from build123d import *

# Parameters (mm, degrees)
SCHIZZO1_R                   = 3.5
ESTRUSIONE_ESTRUSIONE1_DEPTH = 3
ESTRUSIONE_ESTRUSIONE2_DEPTH = 1.5
SCHIZZO3_R                   = 2.5
TAGLIO_ESTRUSIONE1_DEPTH     = 2
RACCORDO1_R                  = 1
SKETCH2_R                    = 1
CUT_EXTRUDE1_DEPTH           = 17.046806536


with BuildPart() as part:
    # Schizzo1 → Estrusione-Estrusione1 (new body)
    with BuildSketch(Plane(origin=(0, 0, 0), x_dir=(1, 0, 0), z_dir=(0, 1, 0))):
        with Locations(Location((0, 0, 0), (0, 0, 270))):
            Circle(SCHIZZO1_R)
    extrude(amount=ESTRUSIONE_ESTRUSIONE1_DEPTH)

    # Schizzo2 → Estrusione-Estrusione2 (add)
    with BuildSketch(Plane(origin=(0, 3, 0), x_dir=(1, 0, 0), z_dir=(0, 1, 0))):
        with BuildLine():
            Line((15, 1.5), (15, -1.5))
            Line((15, -1.5), (0.469834495, -3.468321719))
            ThreePointArc((0.469834495, -3.468321719), (-3.5, 0), (0.469834495, 3.468321719))
            Line((0.469834495, 3.468321719), (15, 1.5))
        make_face()
    extrude(amount=ESTRUSIONE_ESTRUSIONE2_DEPTH)

    # Schizzo3 → Taglio-Estrusione1 (cut)
    with BuildSketch(Plane.XZ):
        with Locations(Location((0, 0, 0), (0, 0, 270))):
            Circle(SCHIZZO3_R)
    extrude(amount=-TAGLIO_ESTRUSIONE1_DEPTH, mode=Mode.SUBTRACT)

    # Raccordo1
    raccordo1_edges = [part.edges().sort_by_distance(p)[0] for p in [
        (15, 3.75, 1.5),
        (15, 3.75, -1.5),
    ]]
    fillet(raccordo1_edges, radius=RACCORDO1_R)

    # Sketch2 → Cut-Extrude1 (cut, through all)
    with BuildSketch(Plane(origin=(0, 4.5, 0), x_dir=(1, 0, 0), z_dir=(0, 1, 0))):
        with Locations(Location((13, 0.055401887, 0), (0, 0, 270))):
            Circle(SKETCH2_R)
    extrude(amount=-CUT_EXTRUDE1_DEPTH, mode=Mode.SUBTRACT)


solid = part.part
Work out the finished part from the listing and answer in its coordinate system (mm). A direction names the side the tool comes from. Round coordinates to 2 decimals unless told otherwise and drop trailing zeros. Write each loop counter-clockwise with the first axis right and the second up, starting at its lowest first coordinate (ties: lowest second). Pieces come first, ordered by that corner, then holes. Notation, with made-up numbers: M 68,-5 L 114,-5 A22 ccw 114,24 Z; hole C 65,3.5 d11. An arc over 180 degrees is marked long. Use a Markdown table: item, result.
1) Which of the six approach directions +Z, -Z, +X, -X, +Y, -Y give full straight-line access (tool end or side, diameter ignored) to faces 1 (the face through (4, 4.5, 0)), 2 (the face through (-2.44, 0.99, 0.54))?
Taken from the geometry:
| item | result |
|---|---|
| face 1 | +Z, -Z, +X, -X, +Y |
| face 2 | -Y |
2) The part is cut by section A-A on z = -0.25. Give the vertices of the cut face in (x, y).
Taken from the geometry:
| item | result |
|---|---|
| outline | M -3.49,0 L -2.49,0 L -2.49,2 L 2.49,2 L 2.49,0 L 3.49,0 L 3.49,3 L 12.02,3 L 12.02,4.5 L -3.49,4.5 Z; M 13.98,3 L 15,3 L 15,4.5 L 13.98,4.5 Z |
3) The part is cut by section C-C on y = 1.1. Give the vertices of the cut face in (x, z).
Taken from the geometry:
| item | result |
|---|---|
| outline | C 0,0 d7; hole C 0,0 d5 |
4) Determine the mould class of faces 3 (the face through (7.206, 3.74, -2.556)), 4 (the face through (-2, 0, 2)), 5 (the face through (0, 2, 0)) for opening direction Z: pulls with the +Z half, pulls with the -Z half, needs draft (parallel to the pull), parting line crosses it, or undercut.
Taken from the geometry:
| item | result |
|---|---|
| face 3 | pulls with the -Z half |
| face 4 | needs draft |
| face 5 | undercut |
5) A flat-ended cylindrical pin translates along its axis: pin 1 (2.5 mm diameter, centred on x = 13, z = -0.06, fed in from -Y). Find the tip coordinate at first contact, or state that the pin passes through.
Taken from the geometry:
| item | result |
|---|---|
| pin 1 | stops at y = 3 |
6) The part is cut by section D-D on x = 13. Give the vertices of the cut face in (y, z).
Taken from the geometry:
| item | result |
|---|---|
| outline | M 3,-1.77 L 4.5,-1.77 L 4.5,-1.06 L 3,-1.06 Z; M 3,0.94 L 4.5,0.94 L 4.5,1.77 L 3,1.77 Z |
7) Consider line 1 (X direction, y = 1.4, z = 0); line 2 (Y direction, x = 7.5, z = 0.5); line 3 (Z direction, x = 0.5, y = 3). Determine where each line is inside the solid, lowest interval first. Write a range as [from, to].
Taken from the geometry:
| item | result |
|---|---|
| line 1 | x = [-3.5, -2.5], [2.5, 3.5] |
| line 2 | y = [3, 4.5] |
| line 3 | z = [-3.46, 3.46] |
8) The part is cut by section B-B on x = 0. Give the vertices of the cut face in (y, z), plus the area to 3 significant figures.
Taken from the geometry:
| item | result |
|---|---|
| outline | M 0,-3.5 L 4.5,-3.5 L 4.5,3.5 L 0,3.5 L 0,2.5 L 2,2.5 L 2,-2.5 L 0,-2.5 Z |
| area | 21.5 mm2 |
